The drawing under review shows one solid part. Ordinate dimensions are in mm from its lowest x, y, z. Round coordinates to 2 decimals unless told otherwise and drop trailing zeros. Order: outer loops, then holes, each group sorted by start corner. A loop starts at its lowest first (then second) coordinate and runs counter-clockwise, first axis right, second up. Notation, with made-up numbers: (35.25, 45.25) - (70.25, 45.25) arc R13 cw to (70.25, 62.25) - close; hole circle Ø9 at (3.5, 66.5). An arc over 180 degrees is marked (long way). Answer as a JSON object with one key per item and string values. Group by question number.
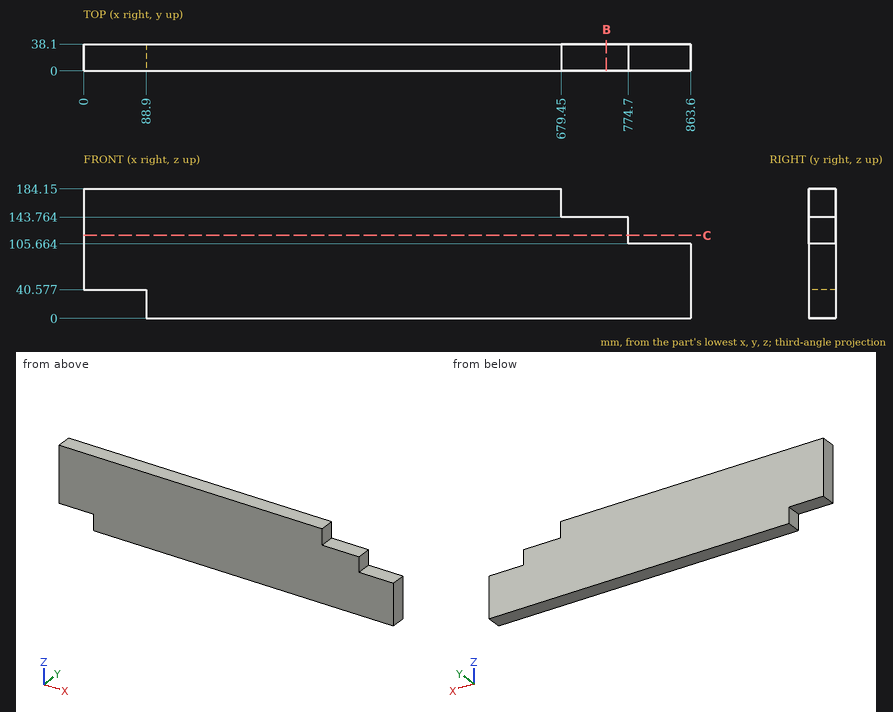
1. Take a section at C-C, the plane z = 118. Give the boundary of the cut face in (x, y).
2. To check wall thickness, follow line 1 (Z direction, x = 768.5, y = 2.5) (1 decimal); line 2 (Z direction, x = 43, y = 10); line 3 (X direction, y = 5, z = 154.5). State the ranges of each line that lie inside material, in increasing order. Write a range as from..to.
3. Clearance check with flat-ended pins moving along their axes: P1, Ø6, axis at x = 208.5, z = 65, coming from the -Y side; P2, Ø19, axis at x = 43, y = 18, coming from the -Z side; P3, Ø11.5, axis at y = 26.5, z = 119.5, coming from the +X side; P4, Ø11.5, axis at y = 17, z = 163, coming from the +X side. State where each tip first meets the part, or that it passes through.
4. Take a section at B-B, the plane x = 743.5. Give the boundary of the cut face in (y, z) (1 decimal).
Response values:
{
 "1": {"outline": "(0, 0) - (774.7, 0) - (774.7, 38.1) - (0, 38.1) - close"},
 "2": {"line 1": "0..143.8", "line 2": "40.58..184.15", "line 3": "0..679.45"},
 "3": {"P1": "y = 0", "P2": "z = 40.58", "P3": "x = 774.7", "P4": "x = 679.45"},
 "4": {"outline": "(0, 0) - (38.1, 0) - (38.1, 143.8) - (0, 143.8) - close"}
}
